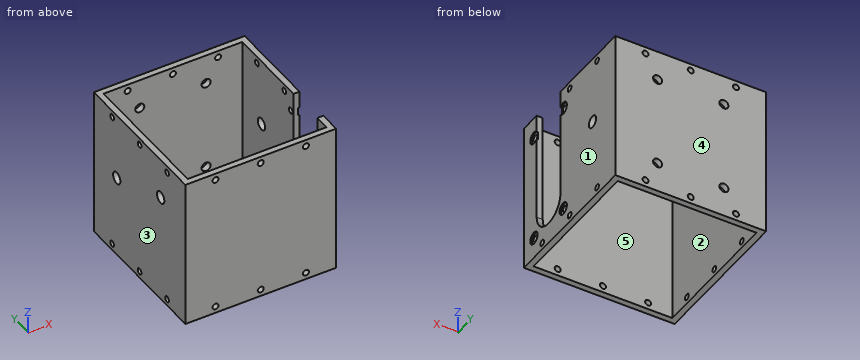
Autodesk Inventor part; units mm, degrees
ref_plane "YZ Plane" through (0, 0, 0) normal (1, 0, 0) x (0, 1, 0)
ref_plane "XZ Plane" through (0, 0, 0) normal (0, 1, 0) x (-1, 0, 0)
ref_plane "XY Plane" through (0, 0, 0) normal (0, 0, 1) x (1, 0, 0)
sketch "スケッチ1" plane through (0, 0, 0) normal (0, 0, 1) x (1, 0, 0)
  line L0 (-25, 25) -> (25, 25)
  line L1 (25, 25) -> (25, -25)
  line L2 (25, -25) -> (-25, -25)
  line L3 (-25, -25) -> (-25, 25)
  line L4 (-23, 23) -> (23, 23)
  line L5 (23, 23) -> (23, -23)
  line L6 (23, -23) -> (-23, -23)
  line L7 (-23, -23) -> (-23, 23)
  point P0 (0, 0)
  dimension "d0" = 50
  dimension "d1" = 50
  dimension "d4" = 25
  dimension "d5" = 25
  dimension "d6" = 46
  dimension "d7" = 2
  dimension "d8" = 46
  dimension "d9" = 2
extrude "押し出し1" add sketch "スケッチ1" along normal blind 50
sketch "スケッチ2" plane through (25, -25, 0) normal (1, 0, 0) x (0, 0, -1)
  line L0 (-50, 50) -> (-50, 0)
  line L1 (0, 0) -> (-50, 0)
  line L2 (-50, 20) -> (-13.5, 20)
  line L3 (-13.5, 7) -> (-50, 7)
  line L4 (-50, 7) -> (-50, 20)
  arc A0 (-13.5, 7) -> (-13.5, 20) centre (-13.5, 13.5) ccw
  point P0 (0, 25)
  point P1 (-7, 13.5)
  dimension "d34" = 13
  dimension "d35" = 7
  dimension "d43" = 13
  dimension "d44" = 6.5
  dimension "d46" = 36.5
extrude "押し出し2" cut sketch "スケッチ2" against normal blind 30.5
sketch "スケッチ3" plane through (25, -25, 0) normal (1, 0, 0) x (0, 0, -1)
  arc A0 (-13.5, 7) -> (-13.5, 20) centre (-13.5, 13.5) ccw
  line L0 (-13.5, 7) -> (-50, 7)
  circle A1 centre (-7, 21.5) radius 1
  circle A2 centre (-43, 21.5) radius 1
  circle A3 centre (-43, 5.5) radius 1
  circle A4 centre (-7, 5.5) radius 1
  point P0 (0, 25)
  dimension "d47" = 8
  dimension "d48" = 8
  dimension "d49" = 16
  dimension "d50" = 1.5
  dimension "d51" = 36
  dimension "d52" = 36
  dimension "d53" = 6.5
  dimension "d55" = 2
  dimension "d56" = 6.5
hole "穴1" at (25, -19.5, 43) at (25, -3.5, 7) at (25, -19.5, 7) at (25, -3.5, 43) direction (-1, 0, 0) diameter 2 depth 2 tip angle 118 counterbore diameter 4 counterbore depth 0.5
sketch "スケッチ11" plane through (25, -25, 0) normal (1, 0, 0) x (0, 0, -1)
  line L0 (0, 0) -> (-50, 0)
  circle A0 centre (-27.5, 37.5) radius 1.5
  line L1 (-50, 50) -> (-50, 20)
  circle A1 centre (-36.5, 13.5) radius 1.5
  line L2 (0, 50) -> (0, 0)
  point P0 (0, 25)
  dimension "d108" = 13.5
  dimension "d109" = 3
  dimension "d110" = 13.5
  dimension "d128" = 24
  dimension "d137" = 27.5
hole "穴6" at (25, -11.5, 36.5) at (25, 12.5, 27.5) direction (-1, 0, 0) diameter 4 end through all
sketch "スケッチ15" plane through (-25, -25, 0) normal (0, -1, 0) x (1, 0, 0)
  line L0 (50, 50) -> (0, 50)
  line L1 (0, 0) -> (0, 50)
  circle A0 centre (10, 47.75) radius 1
  circle A1 centre (25, 47.75) radius 1
  circle A2 centre (40, 47.75) radius 1
  line L2 (50, 0) -> (0, 0)
  circle A3 centre (10, 2.25) radius 1
  circle A4 centre (25, 2.25) radius 1
  circle A5 centre (40, 2.25) radius 1
  point P0 (49.5, 0)
  point P1 (49.5, 50)
  point P2 (25, 0)
  dimension "d138" = 2
  dimension "d139" = 10
  dimension "d141" = 2.25
  dimension "d142" = 2.25
  dimension "d143" = 2.25
  dimension "d144" = 15
  dimension "d166" = 15
  dimension "d167" = 10
  dimension "d168" = 15
  dimension "d169" = 15
  dimension "d170" = 2.25
  dimension "d171" = 2.25
  dimension "d172" = 2.25
hole "穴10" at (-15, -25, 47.75) at (-15, -25, 2.25) at (0, -25, 47.75) at (0, -25, 2.25) at (15, -25, 2.25) at (15, -25, 47.75) direction (0, 1, 0) diameter 2 end through all
sketch "スケッチ16" plane through (-25, -25, 0) normal (-1, 0, 0) x (0, 0, 1)
  line L0 (50, 0) -> (50, 50)
  line L1 (0, 50) -> (50, 50)
  line L2 (0, 0) -> (50, 0)
  circle A0 centre (47.75, 40) radius 1
  circle A1 centre (47.75, 25) radius 1
  circle A2 centre (47.75, 10) radius 1
  circle A3 centre (2.25, 40) radius 1
  circle A4 centre (2.25, 25) radius 1
  circle A5 centre (2.25, 10) radius 1
  line L3 (0, 48) -> (0, 2)
  point P0 (0, 25)
  dimension "d152" = 2
  dimension "d153" = 2.25
  dimension "d154" = 2.25
  dimension "d155" = 2.25
  dimension "d156" = 10
  dimension "d157" = 10
  dimension "d158" = 15
  dimension "d173" = 15
  dimension "d174" = 15
  dimension "d175" = 10
  dimension "d176" = 2.25
  dimension "d177" = 2.25
  dimension "d178" = 2.25
hole "穴11" at (-25, 15, 2.25) at (-25, 0, 2.25) at (-25, -15, 2.25) at (-25, -15, 47.75) at (-25, 0, 47.75) at (-25, 15, 47.75) direction (1, 0, 0) diameter 2 end through all
sketch "スケッチ17" plane through (-25, 25, 50) normal (0, 1, 0) x (1, 0, 0)
  circle A0 centre (25, 2.25) radius 1
  line L0 (0, 50) -> (50, 50)
  line L1 (0, 0) -> (50, 0)
  circle A1 centre (14, 40) radius 1.5
  circle A2 centre (36, 40) radius 1.5
  circle A3 centre (14, 10) radius 1.5
  circle A4 centre (36, 10) radius 1.5
  point P0 (49.5, 0)
  point P1 (49.5, 50)
  point P2 (25, 50)
  dimension "d196" = 3
  dimension "d197" = 11
  dimension "d198" = 11
  dimension "d199" = 10
  dimension "d200" = 10
  dimension "d201" = 10
  dimension "d202" = 10
  dimension "d203" = 11
  dimension "d204" = 11
hole "穴12" at (11, 25, 40) at (-11, 25, 40) at (11, 25, 10) at (-11, 25, 10) direction (0, -1, 0) diameter 3 depth 2 tip angle 118
thread "ねじ1"
thread "ねじ2"
thread "ねじ3"
thread "ねじ4"
properties material "アルミニウム 6061"
The model under review builds one solid part; all positions refer to its coordinate system, in mm. Face numbers are marked on the shaded views. A direction names the side the tool comes from. Coordinates: 2 decimals unless noted, no trailing zeros. Order: outer loops, then holes, each group sorted by start corner. A loop starts at its lowest first (then second) coordinate and runs counter-clockwise, first axis right, second up. Notation, with made-up numbers: (-2, 79.25) -> (14, 79.25) arc R11 ccw to (14, 83.25) -> close; hole circle Ø11 at (-1.5, -37.75). An arc over 180 degrees is marked (long way). Answer in a Markdown table with one row per item.
(1) Machinability: for the marked faces 1 and 2, which of the approach directions +Z, -Z, +X, -X, +Y, -Y give a long, thin tool a straight path to every point of the face, cutting with its end or side? Answer none if there is none.
Answers:
| item | result |
|---|---|
| face 1 | +Z, -Z, +X, +Y, -Y |
| face 2 | +Z, -Z |
(2) Wall thickness on line 1 along Z through (x, y) = (-11, 24.4); line 2 along X through (y, z) = (24.4, 2.25); line 3 along Z through (x, y) = (0, -23.8): over which ranges is each line inside the solid? List them lowest first.
Answers:
| item | result |
|---|---|
| line 1 | 0 to 8.5, 11.5 to 38.5, 41.5 to 50 |
| line 2 | -25 to -16, -14 to -1, 1 to 14, 16 to 25 |
| line 3 | 0 to 1.25, 3.25 to 46.75, 48.75 to 50 |
(3) The part is to be moulded in two halves that separate along Y. For the marked faces 3, 4 and 5, say which applies: +Y half, -Y half, draft (parallel to the pull), parting line (faces both ways), or undercut.
Answers:
| item | result |
|---|---|
| face 3 | draft |
| face 4 | +Y half |
| face 5 | undercut |
(4) Consider section B-B (y = -11.5). Write out the cut boundary in (x, z), plus the area to 3 significant figures.
Answers:
| item | result |
|---|---|
| outline | (-25, 0) -> (-23, 0) -> (-23, 34.5) -> (-25, 34.5) -> close; (-25, 38.5) -> (-23, 38.5) -> (-23, 50) -> (-25, 50) -> close; (23, 0) -> (25, 0) -> (25, 7) -> (23, 7) -> close |
| area | 106 mm² |
(5) Consider section A-A (z = 27.5). Write out the cut boundary in (x, y), plus the area to 3 significant figures.
Answers:
| item | result |
|---|---|
| outline | (-25, -25) -> (25, -25) -> (25, -18) -> (23, -18) -> (23, -23) -> (-23, -23) -> (-23, 10.5) -> (-25, 10.5) -> close; (-25, 14.5) -> (-23, 14.5) -> (-23, 23) -> (23, 23) -> (23, 14.5) -> (25, 14.5) -> (25, 25) -> (-25, 25) -> close; (23, -5) -> (25, -5) -> (25, 10.5) -> (23, 10.5) -> close |
| area | 342 mm² |
(6) Consider section C-C (x = 0). Write out the cut boundary in (y, z), plus the area to 3 significant figures.
Answers:
| item | result |
|---|---|
| outline | (-25, 0) -> (-23, 0) -> (-23, 1.25) -> (-25, 1.25) -> close; (-25, 3.25) -> (-23, 3.25) -> (-23, 46.75) -> (-25, 46.75) -> close; (-25, 48.75) -> (-23, 48.75) -> (-23, 50) -> (-25, 50) -> close; (23, 0) -> (25, 0) -> (25, 1.25) -> (23, 1.25) -> close; (23, 3.25) -> (25, 3.25) -> (25, 46.75) -> (23, 46.75) -> close; (23, 48.75) -> (25, 48.75) -> (25, 50) -> (23, 50) -> close |
| area | 184 mm² |
(7) Insertion check: pin 1 (3 mm diameter, centred on y = -19, z = 7.5, fed in from +X); pin 2 (1.2 mm diameter, centred on y = 15, z = 2.25, fed in from +X) (1 decimal). Each pin has a flat end and moves straight along its axis. Give the tip position at first contact, or say it passes through.
Answers:
| item | result |
|---|---|
| pin 1 | x = 25 |
| pin 2 | through |
